The listing builds one solid part. Answer for the finished solid, in the listing's coordinates (mm). Give positions to 0.01 mm unless a question says otherwise; leave off trailing zeros. Order: outer loops, then holes, each group sorted by start corner. A loop starts at its lowest first (then second) coordinate and runs counter-clockwise, first axis right, second up. Notation, with made-up numbers: (36, 1) - (83, 1) arc R21 ccw to (83, 25) - close; hole circle Ø2 at (34.25, -11.5). An arc over 180 degrees is marked (long way). Answer as a JSON object with one key per item and string values. Group by question number.
Q1. A cutting plane is placed at B-B, the plane x = 70. Give the vertices of the cut face in (y, z), and give its area (3 significant figures).
Q2. Consider line 1 (Z direction, x = 217.5, y = 13.5); line 2 (Y direction, x = 606, z = -93.5). Determine where each line is inside the solid, lowest interval first.
Q3. The mould has two halves that part along Z. Classify faces 1 (the face through (404, 0, -93)), 2 (the face through (404, 8.5, -93)): released by +Z, released by -Z, zero draft, split by the parting line, or undercut.
Q4. Given pin 1 (6 mm diameter, centred on x = 258.5, z = -109.5, fed in from +Y), flat-ended and moving along its own axis, determine where the tip first touches the part or whether it passes through.
Q5. A cutting plane is placed at A-A, the plane y = 13. Give the vertices of the cut face in (x, z), and give its area (3 significant figures).
Q6. A cutting plane is placed at C-C, the plane z = -101.5. Give the vertices of the cut face in (x, y), and give its area (4 significant figures).
from build123d import *

# Parameters (mm, degrees)
SKETCH_1_W          = 1000
SKETCH_1_H          = 60
EXTRUDE_1_DEPTH     = 15
SKETCH_2_W          = 1000
SKETCH_2_H          = 50
CUT_EXTRUDE_1_DEPTH = 10
SCALE_1_SCALE       = 1.7


with BuildPart() as part:
    # 草图1 → 凸台-拉伸1 (new body)
    with BuildSketch(Plane(origin=(0, 0, 0), x_dir=(1, 0, 0), z_dir=(0, 1, 0))):
        with Locations((244.680851064, 54.219858156)):
            Rectangle(SKETCH_1_W, SKETCH_1_H)
    extrude(amount=EXTRUDE_1_DEPTH)

    # 草图2 → 切除-拉伸1 (cut)
    with BuildSketch(Plane(origin=(0, 15, 0), x_dir=(1, 0, 0), z_dir=(0, 1, 0))):
        with Locations((244.680851064, 54.219858156)):
            Rectangle(SKETCH_2_W, SKETCH_2_H)
    extrude(amount=-CUT_EXTRUDE_1_DEPTH, mode=Mode.SUBTRACT)


with BuildPart() as part_1:
    # 缩放比例1: scaled about (0, 0, 0)
    add(part.part.scale(SCALE_1_SCALE))


solid = part_1.part
Reply:
{
 "1": {"outline": "(0, -143.17) - (25.5, -143.17) - (25.5, -134.67) - (8.5, -134.67) - (8.5, -49.67) - (25.5, -49.67) - (25.5, -41.17) - (0, -41.17) - close", "area": "1,160 mm^2"},
 "2": {"line 1": "z = -143.17 to -134.67, -49.67 to -41.17", "line 2": "y = 0 to 8.5"},
 "3": {"face 1": "zero draft", "face 2": "undercut"},
 "4": {"pin 1": "stops at y = 8.5"},
 "5": {"outline": "(-434.04, -143.17) - (1265.96, -143.17) - (1265.96, -134.67) - (-434.04, -134.67) - close; (-434.04, -49.67) - (1265.96, -49.67) - (1265.96, -41.17) - (-434.04, -41.17) - close", "area": "28,900 mm^2"},
 "6": {"outline": "(-434.04, 0) - (1265.96, 0) - (1265.96, 8.5) - (-434.04, 8.5) - close", "area": "14,450 mm^2"}
}
